Part model, mm, in its own coordinate system. Round coordinates to 2 decimals unless told otherwise and drop trailing zeros. Loops run counter-clockwise (first coordinate to the right, second up) from the corner with the lowest first, then second, coordinate; pieces in that order, holes last.
(1) Cut at B-B on z = 4.5. List the corners of the cut face in (x, y) (3 decimals), then the cut area to 3 significant figures.
(2) Probe probe 1 along X at (y, z) = (1.9, 18); probe 2 along X at (y, z) = (0.5, 16); probe 3 along X at (y, z) = (2.4, 8). List the from-to ranges inside material, lowest first.
(3) Cut at D-D on z = -44.5. List the corners of the cut face in (x, y).
(4) Cut at A-A on x = -5. List the corners of the cut face in (y, z), then the cut area to 3 significant figures.
(5) Cut at C-C on y = 2.1. Count the separate pieces of the cut face and the enclosed holes in it, then the cut area to 3 significant figures.
(6) Flat gauge pins, fed straight in: pin 1 (0.9 mm diameter, centred on y = 2, z = -0.5, fed in from +X); pin 2 (4 mm diameter, centred on x = -13.5, z = -7.79, fed in from -Y). Where does each tip first touch, or does it go through?
from build123d import *

# Parameters (mm, degrees)
SKETCH1_R           = 2.25
SKETCH1_R_2         = 11
SKETCH1_R_3         = 3
BOSS_EXTRUDE1_DEPTH = 2.9


with BuildPart() as part:
    # Sketch1 → Boss-Extrude1 (new body)
    with BuildSketch(Plane(origin=(0, 0, 0), x_dir=(1, 0, 0), z_dir=(0, 1, 0))):
        with BuildLine():
            ThreePointArc((-23.5, -19.918584287), (-25.801559897, -26.651870244), (-31.743116322, -30.567508758))
            Line((-31.743116322, -30.567508758), (-13.784418389, -25.918209071))
            ThreePointArc((-13.784418389, -25.918209071), (0, -24.162831426), (13.784418389, -25.918209071))
            Line((13.784418389, -25.918209071), (31.743116322, -30.567508758))
            ThreePointArc((31.743116322, -30.567508758), (24.973720558, -14.418584287), (42.343797276, -12.206590751))
            Line((42.343797276, -12.206590751), (29.338036671, 1.021448035))
            ThreePointArc((29.338036671, 1.021448035), (20.925625842, 12.081415713), (15.553618282, 24.896761037))
            Line((15.553618282, 24.896761037), (10.600680954, 42.774099509))
            ThreePointArc((10.600680954, 42.774099509), (10.899713081, 41.319145212), (11, 39.837168574))
            ThreePointArc((11, 39.837168574), (-1.481976638, 28.937455493), (-10.600680954, 42.774099509))
            Line((-10.600680954, 42.774099509), (-15.553618282, 24.896761037))
            ThreePointArc((-15.553618282, 24.896761037), (-20.925625842, 12.081415713), (-29.338036671, 1.021448035))
            Line((-29.338036671, 1.021448035), (-42.343797276, -12.206590751))
            ThreePointArc((-42.343797276, -12.206590751), (-30.333572876, -9.738167546), (-23.5, -19.918584287))
        make_face()
        with Locations((0, -15.588457268)):
            Circle(SKETCH1_R, mode=Mode.SUBTRACT)
        with Locations((-13.5, 7.794228634)):
            Circle(SKETCH1_R, mode=Mode.SUBTRACT)
        with BuildLine():
            Line((-9.625, -5.578978401), (-9.625, 5.578978401))
            ThreePointArc((-9.625, 5.578978401), (0, 11.125), (9.625, 5.578978401))
            Line((9.625, 5.578978401), (9.625, -5.578978401))
            ThreePointArc((9.625, -5.578978401), (0, -11.125), (-9.625, -5.578978401))
        make_face(mode=Mode.SUBTRACT)
        with Locations((13.5, 7.794228634)):
            Circle(SKETCH1_R, mode=Mode.SUBTRACT)
        with Locations((-34.5, -19.918584287)):
            Circle(SKETCH1_R_2)
        with Locations((-34.5, -19.918584287)):
            Circle(SKETCH1_R_3, mode=Mode.SUBTRACT)
        with Locations((34.5, -19.918584287)):
            Circle(SKETCH1_R_2)
        with Locations((34.5, -19.918584287)):
            Circle(SKETCH1_R_3, mode=Mode.SUBTRACT)
        with Locations((0, 39.837168574)):
            Circle(SKETCH1_R_2)
        with Locations((0, 39.837168574)):
            Circle(SKETCH1_R_3, mode=Mode.SUBTRACT)
    extrude(amount=BOSS_EXTRUDE1_DEPTH)


solid = part.part
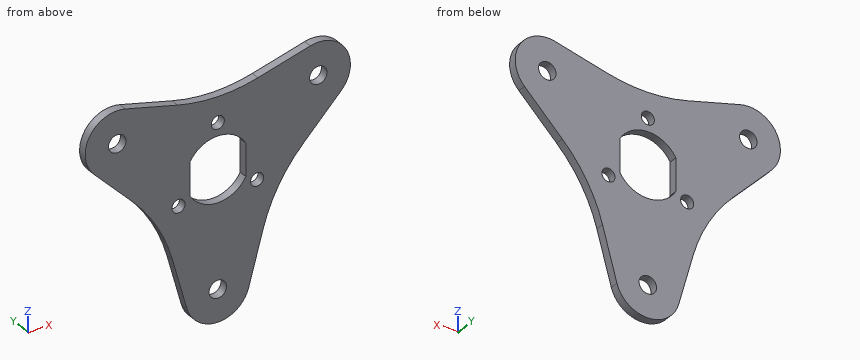
Final values:
1. outline: (-34.767, 0) - (-9.625, 0) - (-9.625, 2.9) - (-34.767, 2.9) - close; (9.625, 0) - (34.767, 0) - (34.767, 2.9) - (9.625, 2.9) - close
1. area: 146 mm2
2. probe 1: x = -45.33 to -36.81, -32.19 to 32.19, 36.81 to 45.33
2. probe 2: x = -44.78 to -2.21, 2.21 to 44.78
2. probe 3: x = -38.21 to -7.73, 7.73 to 38.21
3. outline: (-9.96, 0) - (9.96, 0) - (9.96, 2.9) - (-9.96, 2.9) - close
4. outline: (0, -49.64) - (2.9, -49.64) - (2.9, -9.94) - (0, -9.94) - close; (0, 9.94) - (2.9, 9.94) - (2.9, 24.39) - (0, 24.39) - close
4. area: 157 mm2
5. separate pieces: 1
5. enclosed holes: 7
5. area: 3,420 mm2
6. pin 1: stops at x = 30.29
6. pin 2: passes through
